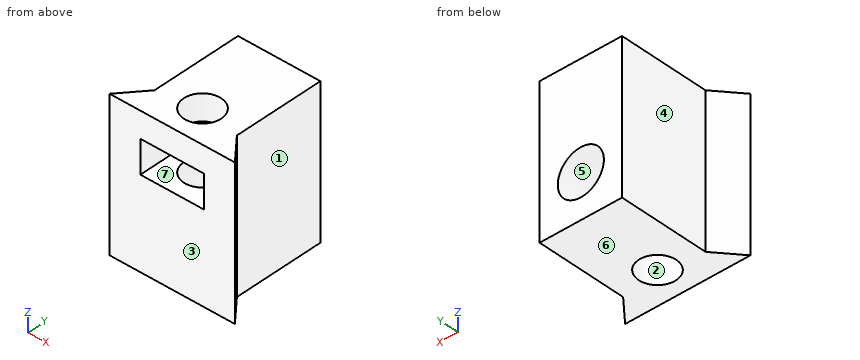
```python
from build123d import *

# Parameters (mm, degrees)
CROQUIS1_R                 = 1.7
SALIENTE_EXTRUIR1_DEPTH    = 13.5
CROQUIS2_R                 = 2.1
CORTAR_EXTRUIR1_DEPTH      = 5.1
CORTAR_EXTRUIR2_DEPTH      = 1.5
CORTAR_EXTRUIR2_DEPTH_BACK = 1.5


with BuildPart() as part:
    # Croquis1 → Saliente-Extruir1 (new body)
    with BuildSketch(Plane.XY):
        Polygon((-5.7, 0), (5.7, 0), (3.75, 2.323919506), (3.75, 10.6), (-3.75, 10.6), (-3.75, 2.323919506), align=None)
        with Locations((0, 3)):
            Circle(CROQUIS1_R, mode=Mode.SUBTRACT)
    extrude(amount=SALIENTE_EXTRUIR1_DEPTH)

    # Croquis2 → Cortar-Extruir1 (cut)
    with BuildSketch(Plane(origin=(0, 10.6, 0), x_dir=(1, 0, 0), z_dir=(0, 1, 0))):
        with Locations((0, -4)):
            Circle(CROQUIS2_R)
    extrude(amount=-CORTAR_EXTRUIR1_DEPTH, mode=Mode.SUBTRACT)

    # Croquis3 → Cortar-Extruir2 (cut, two sides)
    with BuildSketch(Plane.XY.offset(9.65)) as cortar_extruir2_sk:
        Polygon((-2.901185103, 1.325), (-2.901185103, -5.325), (2.901185103, -5.325), (2.901185103, 1.325), (2.901185103, 4.675), (0, 6.35), (-2.901185103, 4.675), align=None)
    extrude(amount=CORTAR_EXTRUIR2_DEPTH, mode=Mode.SUBTRACT)
    extrude(cortar_extruir2_sk.sketch, amount=-CORTAR_EXTRUIR2_DEPTH_BACK, mode=Mode.SUBTRACT)


solid = part.part
```
Can you work these out from the model? Positions are in its coordinate system, mm. Face numbers are marked on the shaded views. A direction names the side the tool comes from. Give positions to 0.01 mm unless a question says otherwise; leave off trailing zeros. Order: outer loops, then holes, each group sorted by start corner. A loop starts at its lowest first (then second) coordinate and runs counter-clockwise, first axis right, second up. Notation, with made-up numbers: M 50,13 L 63,13 A30 ccw 63,38 Z; hole C -15.5,64 d6. An arc over 180 degrees is marked long. Write item = value, one per line. Start each with the question number.
Q1. We'd pull the mould along X, two halves only. Please class the marked faces 1, 2 and 3: pulls with the +X half, pulls with the -X half, needs draft (parallel to the pull), parting line crosses it, or undercut.
Q2. I need wall thicknesses on probe 1 along Y at (x, z) = (0, 11.8); probe 2 along Z at (x, y) = (0, 9.5); probe 3 along X at (y, z) = (3, 6.5). Which ranges of each line are inside material? Lowest first, please. Write a range as [from, to].
Q3. Suppose I cut it at B-B (z = 7.25). Write out the boundary of the cut face in (x, y).
Q4. For the marked faces 4, 5, 6 and 7, which set-ups out of +Z, -Z, +X, -X, +Y, -Y let a thin tool reach every point of the face, with its end or its side?
Q5. Will these pins go through, and if not, where does the flat tip stop? pin 1 Ø2.5 at (x, y) = (0, 3) entering from -Z; pin 2 Ø3.5 at (y, z) = (3.5, 9.5) entering from +X; pin 3 Ø3 at (x, z) = (2, 3) entering from -Y; pin 4 Ø2.5 at (y, z) = (6, 5.5) entering from -X.
Q6. Suppose I cut it at A-A (y = 3). Write out the boundary of the cut face in (x, z).
Q7. Suppose I cut it at C-C (x = 1.5). Write out the boundary of the cut face in (y, z).
Q8. Suppose I cut it at D-D (y = 7). Write out the boundary of the cut face in (x, z).
Check result:
q1.face_1 = pulls with the +X half
q1.face_2 = undercut
q1.face_3 = needs draft
q2.probe_1 = [0, 1.3], [4.7, 10.6]
q2.probe_2 = [0, 1.9], [6.1, 13.5]
q2.probe_3 = [-3.75, -1.7], [1.7, 3.75]
q3.outline = M -5.7,0 L 5.7,0 L 3.75,2.32 L 3.75,10.6 L -3.75,10.6 L -3.75,2.32 Z; hole C 0,3 d3.4
q4.face_4 = +Z, -Z, -X, +Y
q4.face_5 = +Y
q4.face_6 = -Z, +X, -X, +Y, -Y
q4.face_7 = -Y
q5.pin_1 = through
q5.pin_2 = 4.23
q5.pin_3 = 0
q5.pin_4 = -3.75
q6.outline = M -3.75,0 L -1.7,0 L -1.7,8.15 L -2.9,8.15 L -2.9,11.15 L -1.7,11.15 L -1.7,13.5 L -3.75,13.5 Z; M 1.7,0 L 3.75,0 L 3.75,13.5 L 1.7,13.5 L 1.7,11.15 L 2.9,11.15 L 2.9,8.15 L 1.7,8.15 Z
q7.outline = M 0,0 L 2.2,0 L 2.2,8.15 L 0,8.15 Z; M 0,11.15 L 2.2,11.15 L 2.2,13.5 L 0,13.5 Z; M 3.8,0 L 10.6,0 L 10.6,2.53 L 5.5,2.53 L 5.5,5.47 L 10.6,5.47 L 10.6,13.5 L 3.8,13.5 L 3.8,11.15 L 5.48,11.15 L 5.48,8.15 L 3.8,8.15 Z
q8.outline = M -3.75,0 L 3.75,0 L 3.75,13.5 L -3.75,13.5 Z; hole C 0,4 d4.2
